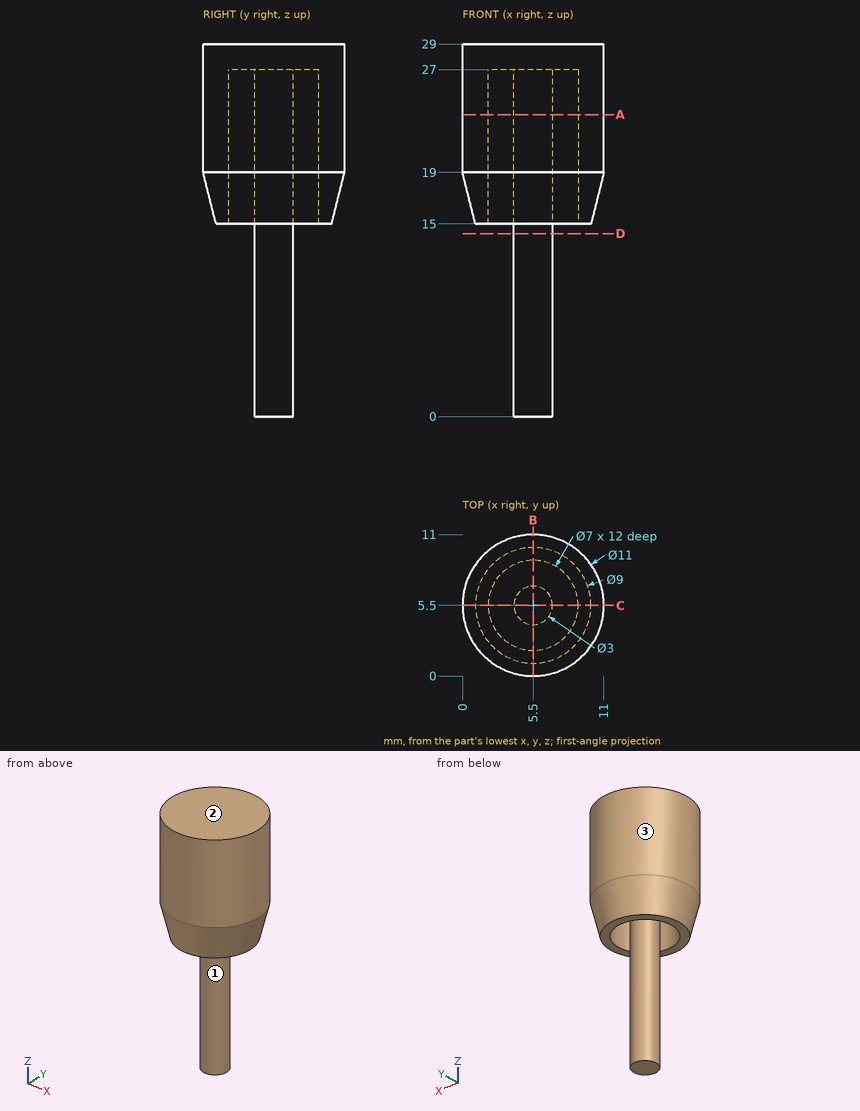
Design review of the part shown in the three views and the two pictorial views. Dimensions are in mm from the part's minimum x, y and z. Give positions to 0.01 mm unless a question says otherwise; leave off trailing zeros. Order: outer loops, then holes, each group sorted by start corner. A loop starts at its lowest first (then second) coordinate and runs counter-clockwise, first axis right, second up. Notation, with made-up numbers: M -31,74 L -14,74 A9 cw -14,89 Z; hole C 8.5,42.5 d7. An arc over 180 degrees is marked long. Answer in a Markdown table with one row per item. Add a question column.
(1) Consider section B-B on x = 5.5. State the section outline as (y, z) points, and give its area (3 significant figures).
(2) For pin 1 (1.5 mm diameter, centred on x = 5, z = 13, fed in from -Y); pin 2 (2 mm diameter, centred on y = 3.5, z = 4.5, fed in from -X); pin 3 (3 mm diameter, centred on y = 7.5, z = 24, fed in from -X), all flat-tipped, find the tip position at first contact; note any pin that passes through.
(3) Consider section D-D on z = 14.25. State the section outline as (x, y) points.
(4) Consider section A-A on z = 23.5. State the section outline as (x, y) points, and give its area (3 significant figures).
(5) Mouldability with a two-part tool opening along Y and no side actions: class the marked faces 1, 2 and 3 as +Y half, -Y half, draft (parallel to the pull), parting line (faces both ways), or undercut.
(6) Wall thickness on probe 1 along Y at (x, z) = (5.5, 20.5); probe 2 along Y at (x, z) = (5.5, 18); probe 3 along Z at (x, y) = (2.25, 7): over which ranges is each line inside the solid? List them lowest first. Write a range as [from, to].
Evaluation:
| question | item | result |
|---|---|---|
| 1 | outline | M 0,19 L 1,15 L 2,15 L 2,27 L 4,27 L 4,0 L 7,0 L 7,27 L 9,27 L 9,15 L 10,15 L 11,19 L 11,29 L 0,29 Z |
| 1 | area | 147 mm^2 |
| 2 | pin 1 | stops at y = 4 |
| 2 | pin 2 | stops at x = 4.38 |
| 2 | pin 3 | stops at x = 0.02 |
| 3 | outline | C 5.5,5.5 d3 |
| 4 | outline | C 5.5,5.5 d11; C 5.5,5.5 d3; hole C 5.5,5.5 d7 |
| 4 | area | 63.6 mm^2 |
| 5 | face 1 | undercut |
| 5 | face 2 | draft |
| 5 | face 3 | parting line |
| 6 | probe 1 | y = [0, 2], [4, 7], [9, 11] |
| 6 | probe 2 | y = [0.25, 2], [4, 7], [9, 10.75] |
| 6 | probe 3 | z = [15, 29] |
